```python
from build123d import *

# Parameters (mm, degrees)
F0_W     = 25.4
F0_H     = 25.4
F0_W_2   = 19.05
F0_H_2   = 19.05
F1_DEPTH = 609.6
F2_W     = 19.05
F2_H     = 19.05
F3_DEPTH = 19.05


with BuildPart() as f1:
    # F0 (on Front) → F1 (new body)
    with BuildSketch(Plane.XZ):
        with Locations((-9.525, 9.525)):
            Rectangle(F0_W, F0_H)
        with Locations((-9.525, 9.525)):
            Rectangle(F0_W_2, F0_H_2, mode=Mode.SUBTRACT)
    extrude(amount=F1_DEPTH)

    # F2 (on face) → F3 (cut)
    with BuildSketch(Plane.XY.offset(22.225)):
        with Locations((-9.525, -304.8)):
            Rectangle(F2_W, F2_H)
    extrude(amount=-F3_DEPTH, mode=Mode.SUBTRACT)


solid = f1.part
```
CAD build for the part. Positions are in the model's coordinates, mm. A direction names the side the tool comes from. Coordinates: 2 decimals unless noted, no trailing zeros. Order: outer loops, then holes, each group sorted by start corner. A loop starts at its lowest first (then second) coordinate and runs counter-clockwise, first axis right, second up. Notation, with made-up numbers: M 69,-1 L 118,-1 A11 cw 118,4 Z; hole C -17,71.5 d1. An arc over 180 degrees is marked long. Write each question's results on one line, items separated by ' | '. Start each with the question number.
Q1. Cut at A-A (y = -367). List the corners of the cut face in (x, z) (3 decimals).
Q2. Which spindle directions (+Z, -Z, +X, -X, +Y, -Y) get a long thin tool onto all of the face, cutting with end or side? Do faces 5 (the flat face through (-10, -460, 19.05)), 6 (the flat face through (-21, -609.6, 10)). Say none if no direction does.
Q3. Cut at B-B (x = -10.25). List the corners of the cut face in (y, z) (3 decimals).
Q4. Flat gauge pin, fed straight in: P1, Ø3, axis at x = -17, z = 16.5, coming from the +Y side. Where does the tip first touch, or does it go through?
Q5. Cut at C-C (z = 8.5). List the corners of the cut face in (x, y) (3 decimals), then the cut area to 3 significant figures.
Q6. Pull direction X, two halves, no side cores. Call faces 1 (the flat face through (0, -309, 11)), 2 (the flat face through (3.175, -301, 9)), 3 (the flat face through (-21, 0, 10)), 4 (the flat face through (-10, -146, 19.05)): +X half, -X half, draft (parallel to the pull), parting line (faces both ways), or undercut.
Q7. Drill centre lines: probe 1 along Z at (x, y) = (-15, -467) (3 decimals); probe 2 along X at (y, z) = (-277, 12) (3 decimals); probe 3 along Y at (x, z) = (-10.5, 20.75) (3 decimals). Where is each one in solid material? Low to high. Write a range as from..to.
Found:
1) outline: M -22.225,-3.175 L 3.175,-3.175 L 3.175,22.225 L -22.225,22.225 Z; hole M -19.05,0 L 0,0 L 0,19.05 L -19.05,19.05 Z
2) face 5: +Y, -Y | face 6: +Z, -Z, +X, -X, -Y
3) outline: M -609.6,-3.175 L 0,-3.175 L 0,0 L -609.6,0 Z; M -609.6,19.05 L -314.325,19.05 L -314.325,22.225 L -609.6,22.225 Z; M -295.275,19.05 L 0,19.05 L 0,22.225 L -295.275,22.225 Z
4) P1: through
5) outline: M -22.225,-609.6 L -19.05,-609.6 L -19.05,0 L -22.225,0 Z; M 0,-609.6 L 3.175,-609.6 L 3.175,0 L 0,0 Z | area: 3,870 mm²
6) face 1: undercut | face 2: +X half | face 3: draft | face 4: undercut
7) probe 1: -3.175..0, 19.05..22.225 | probe 2: -22.225..-19.05, 0..3.175 | probe 3: -609.6..-314.325, -295.275..0
